from build123d import *

# Parameters (mm, degrees)
F1_DEPTH     = 57.15
F0_W         = 21.59
F0_H         = 24.13
F2_DEPTH     = 21.59
F3_DEPTH     = 12.5
F5_R         = 12.5
F6_DEPTH     = 90.806
F7_R         = 20
F8_T         = 2.5
F8_T3_DEPTH  = 107.87
F8_T5_DEPTH  = 14.09
F8_T7_DEPTH  = 29.13
F8_T9_DEPTH  = 14.09
F8_T11_DEPTH = 35.48
F8_T14_ANGLE = 90.000000001
F8_T16_ANGLE = 90.000000001
F8_T18_ANGLE = 180.000000001
F8_T20_ANGLE = 180.000000001


# Not quite as in the source:
# - a shell that OpenCascade refuses in one call is made with other operations: the cavity is built on its own and cut out


with BuildPart() as f1:
    # F0 (on Front) → F1 (new body, symmetric)
    with BuildSketch(Plane.XZ):
        Polygon((-63.5, -9.525), (63.5, -9.525), (63.5, 9.525), (39.37, 9.525), (-63.5, 9.525), align=None)
    extrude(amount=F1_DEPTH, both=True)

    # F0 (on Front) → F2 (join, symmetric)
    with BuildSketch(Plane.XZ):
        with BuildLine():
            Line((39.37, 9.525), (63.5, 9.525))
            Line((63.5, 9.525), (63.5, 40.005))
            ThreePointArc((63.5, 40.005), (65.7318463274, 45.3931536726), (71.12, 47.625))
            Line((71.12, 47.625), (83.82, 47.625))
            Line((83.82, 47.625), (83.82, 71.755))
            Line((83.82, 71.755), (71.12, 71.755))
            ThreePointArc((71.12, 71.755), (48.6693596973, 62.4556403027), (39.37, 40.005))
            Line((39.37, 40.005), (39.37, 9.525))
        make_face()
        with Locations((94.615, 59.69)):
            Rectangle(F0_W, F0_H)
    extrude(amount=F2_DEPTH, both=True)

    # F0 (on Front) → F3 (join, symmetric)
    with BuildSketch(Plane.XZ):
        with BuildLine():
            add(Edge.make_bspline(
                [(-63.5, 9.525), (-63.5, 31.5907289062), (-3.4680848518, 65.1337229979), (32.8965573805, 71.755), (71.12, 71.755)],
                knots=[0, 0, 0, 0, 0.4791248693, 1, 1, 1, 1], degree=3))
            Line((-63.5, 9.525), (39.37, 9.525))
            Line((39.37, 9.525), (39.37, 40.005))
            ThreePointArc((39.37, 40.005), (48.6693596973, 62.4556403027), (71.12, 71.755))
        make_face()
    extrude(amount=F3_DEPTH, both=True)

    # F0 (on Front) → F4 (revolve)
    with BuildSketch(Plane.XZ):
        Polygon((105.41, 81.28), (105.41, 71.755), (105.41, 47.625), (105.41, 38.1), (127, 38.1), (127, 81.28), align=None)
    revolve(axis=Axis((105.41, 0, 59.69), (0, 0, -1)))

    # F5 (on face) → F6 (cut, through all)
    with BuildSketch(Plane.XY.offset(81.28)):
        with Locations((105.41, 0)):
            Circle(F5_R)
    extrude(amount=-F6_DEPTH, mode=Mode.SUBTRACT)

    # F7
    f7_edges = [f1.edges().sort_by_distance(p)[0] for p in [
        (63.5, -57.15, 0),
        (-63.5, -57.15, 0),
        (63.5, 57.15, 0),
        (-63.5, 57.15, 0),
    ]]
    fillet(f7_edges, radius=F7_R)

    # F8: shell of thickness 2.5, made by hand


with BuildPart() as f8_core1:
    # F8_t2: copy of F1
    add(f1.part)

    # the walls: a layer under each face that stays
    f8_faces = [f8_core1.faces().sort_by_distance(p)[0] for p in [
        (0, 57.15, 0),
        (-57.6421356237, 51.2921356237, 0),
        (57.6421356237, 51.2921356237, 0),
        (-63.5, 0, 0),
        (63.5, 0, 15.24),
        (-57.6421356237, -51.2921356237, 0),
        (57.6421356237, -51.2921356237, 0),
        (0, -57.15, 0),
        (0, 34.825, 9.525),
        (0, -34.825, 9.525),
        (-8.3874166975, -6.25, 58.8110273922),
        (-8.3874166975, 6.25, 58.8110273922),
        (50.3766666667, 21.59, 19.8966666667),
        (50.3766666667, -21.59, 19.8966666667),
        (65.7318463274, 0, 45.3931536726),
        (3.81, 12.5, 40.64),
        (39.37, 17.045, 24.765),
        (3.81, -12.5, 40.64),
        (39.37, -17.045, 24.765),
        (88.265, 14.3933333333, 71.755),
        (76.835, 14.3933333333, 47.625),
        (116.205, -18.6974884677, 45.2966666667),
        (48.6693596973, 17.045, 62.4556403027),
        (48.6693596973, -17.045, 62.4556403027),
        (91.0166666667, 14.3933333333, 81.28),
        (119.8033333333, 14.3933333333, 38.1),
        (92.91, 0, 59.69),
    ]]
    thicken(f8_faces, amount=-F8_T, mode=Mode.SUBTRACT)

    # F8_s4 → F8_t3 (cut)
    with BuildSketch(Plane.YZ.offset(-66)):
        Polygon((12.525, 9.55), (12.5, 7.025), (10, 7.025), (10, 9.525), align=None)
        Polygon((-12.525, 9.55), (-12.5, 7.025), (-10, 7.025), (-10, 9.525), align=None)
    extrude(amount=F8_T3_DEPTH, mode=Mode.SUBTRACT)

    # F8_s6 → F8_t5 (cut)
    with BuildSketch(Plane.XZ.offset(-24.09)):
        Polygon((39.345, 9.55), (39.37, 7.025), (41.87, 7.025), (41.87, 9.525), align=None)
    extrude(amount=F8_T5_DEPTH, mode=Mode.SUBTRACT)

    # F8_s8 → F8_t7 (cut)
    with BuildSketch(Plane.YZ.offset(36.87)):
        Polygon((21.615, 9.55), (21.59, 7.025), (19.09, 7.025), (19.09, 9.525), align=None)
        Polygon((-21.615, 9.55), (-21.59, 7.025), (-19.09, 7.025), (-19.09, 9.525), align=None)
    extrude(amount=F8_T7_DEPTH, mode=Mode.SUBTRACT)

    # F8_s10 → F8_t9 (cut)
    with BuildSketch(Plane.XZ.offset(10)):
        Polygon((39.345, 9.55), (39.37, 7.025), (41.87, 7.025), (41.87, 9.525), align=None)
    extrude(amount=F8_T9_DEPTH, mode=Mode.SUBTRACT)

    # F8_s12 → F8_t11 (cut)
    with BuildSketch(Plane.XY.offset(7.025)):
        Polygon((39.345, 12.525), (39.37, 10), (41.87, 10), (41.87, 12.5), align=None)
        Polygon((39.345, -12.525), (39.37, -10), (41.87, -10), (41.87, -12.5), align=None)
    extrude(amount=F8_T11_DEPTH, mode=Mode.SUBTRACT)

    # F8_s13 → F8_t14 (revolve, cut)
    with BuildSketch(Plane.XY.offset(40.005)):
        Polygon((39.345, 12.525), (39.37, 10), (41.87, 10), (41.87, 12.5), align=None)
    revolve(axis=Axis((71.12, 12.5, 40.005), (0, 1, 0)), revolution_arc=F8_T14_ANGLE, mode=Mode.SUBTRACT)

    # F8_s15 → F8_t16 (revolve, cut)
    with BuildSketch(Plane.XY.offset(40.005)):
        Polygon((39.345, -12.525), (39.37, -10), (41.87, -10), (41.87, -12.5), align=None)
    revolve(axis=Axis((71.12, -12.5, 40.005), (0, 1, 0)), revolution_arc=F8_T16_ANGLE, mode=Mode.SUBTRACT)

    # F8_s17 → F8_t18 (revolve, cut)
    with BuildSketch(Plane.YZ.offset(105.41)):
        Polygon((21.615, 71.78), (21.59, 69.255), (19.09, 69.255), (19.09, 71.755), align=None)
    revolve(axis=Axis((105.41, 0, 71.755), (0, 0, 1)), revolution_arc=F8_T18_ANGLE, mode=Mode.SUBTRACT)

    # F8_s19 → F8_t20 (revolve, cut)
    with BuildSketch(Plane.YZ.offset(105.41)):
        Polygon((21.615, 47.6), (21.59, 50.125), (19.09, 50.125), (19.09, 47.625), align=None)
    revolve(axis=Axis((105.41, 0, 47.625), (0, 0, 1)), revolution_arc=F8_T20_ANGLE, mode=Mode.SUBTRACT)


with BuildPart() as f1_1:
    add(f1.part)

    # what is left inside the walls is the cavity
    f8_cavity = [f8_core1.part.solids().sort_by_distance(p)[0] for p in [
        (0, 18.216667, -9.5),
    ]]
    add(f8_cavity, mode=Mode.SUBTRACT)


solid = f1_1.part
Can you work these out from the model? Positions are in its coordinate system, mm. A direction names the side the tool comes from. Give positions to 0.01 mm unless a question says otherwise; leave off trailing zeros. Loops run counter-clockwise (first coordinate to the right, second up) from the corner with the lowest first, then second, coordinate; pieces in that order, holes last. Notation, with made-up numbers: (72, -14) -> (87, -14) arc R20 cw to (87, 9) -> close; hole circle Ø8 at (41.5, 77.5). An arc over 180 degrees is marked (long way). Return JSON: item names as keys, results as strings.
Q1. I want a section at B-B, the plane y = -25. List the corners of the cut face in (x, z) for me (3 decimals), then the cut area to 3 significant figures.
Checks:
{"outline": "(-63.5, -9.525) -> (-61, -9.525) -> (-61, 7.025) -> (61, 7.025) -> (61, -9.525) -> (63.5, -9.525) -> (63.5, 9.525) -> (-63.5, 9.525) -> close", "area": "400 mm2"}
Q2. I need wall thicknesses on probe 1 along X at (y, z) = (23, 1); probe 2 along Z at (x, y) = (71.5, -11.5) (3 decimals); probe 3 along Z at (x, y) = (111, 16.5). Which ranges of each line are inside material? Lowest first, please.
Checks:
{"probe 1": "x = -63.5 to -61, 61 to 63.5", "probe 2": "z = 47.625 to 50.125, 69.255 to 71.755", "probe 3": "z = 38.1 to 40.6, 78.78 to 81.28"}
Q3. We'd pull the mould along Z, two halves only. Please class faces 5 (the face through (81, 0, 71.755)), 6 (the face through (41.87, 15, 23)), 7 (the face through (63.886, -0.267, 47.082)): released by +Z, released by -Z, zero draft, split by the parting line, or undercut.
Checks:
{"face 5": "released by +Z", "face 6": "zero draft", "face 7": "undercut"}
Q4. For pin 1 Ø6 at (x, y) = (-4.5, 29) entering from -Z (3 decimals); pin 2 Ø18.5 at (x, z) = (67, 27) entering from +Y; pin 3 Ø1.5 at (x, z) = (65.5, 51) entering from -Y; pin 4 Ø22.5 at (x, y) = (105.41, 0) entering from +Z, each with a flat end and sliding along its axis, tell me the tip position at first contact or that it passes through.
Checks:
{"pin 1": "stops at z = 7.025", "pin 2": "stops at y = 21.59", "pin 3": "stops at y = -21.59", "pin 4": "passes through"}
Q5. On a 3-axis mill with a long thin cutter (end or side, diameter ignored), from which of +Z, -Z, +X, -X, +Y, -Y can I reach the whole of each face in a straight line? I mean faces 1 (the face through (5, -12.5, 34)), 2 (the face through (1, -33, 7.025)), 3 (the face through (90.425, 0.66, 59.957)), 4 (the face through (65.67, -0.3, 45.33)). Say none if no direction works.
Checks:
{"face 1": "+Z, -X, -Y", "face 2": "-Z", "face 3": "none", "face 4": "-Z, +Y, -Y"}
Q6. I want a section at A-A, the plane z = -0.5. List the corners of the cut face in (x, y) for me, then the cut area to 3 significant figures.
Checks:
{"outline": "(-63.5, -37.15) arc R20 ccw to (-43.5, -57.15) -> (43.5, -57.15) arc R20 ccw to (63.5, -37.15) -> (63.5, 37.15) arc R20 ccw to (43.5, 57.15) -> (-43.5, 57.15) arc R20 ccw to (-63.5, 37.15) -> close; hole (-61, -37.15) arc R17.5 ccw to (-43.5, -54.65) -> (43.5, -54.65) arc R17.5 ccw to (61, -37.15) -> (61, 37.15) arc R17.5 ccw to (43.5, 54.65) -> (-43.5, 54.65) arc R17.5 ccw to (-61, 37.15) -> close", "area": "1,100 mm2"}
Q7. I want a section at C-C, the plane y = -6. Count the separate pieces of the cut face and the enclosed holes in it, then the cut area to 3 significant figures.
Checks:
{"separate pieces": "2", "enclosed holes": "1", "area": "1,130 mm2"}
